The listing builds one solid part. Answer for the finished solid, in the listing's coordinates (mm). Face numbers are marked on the shaded views. A direction names the side the tool comes from. Coordinates: 2 decimals unless noted, no trailing zeros. Write each loop counter-clockwise with the first axis right and the second up, starting at its lowest first coordinate (ties: lowest second). Pieces come first, ordered by that corner, then holes.
(1) Which of the six approach directions +Z, -Z, +X, -X, +Y, -Y give full straight-line access (tool end or side, diameter ignored) to the marked faces 1, 2 and 3?
(2) Given P1, Ø5.5, axis at x = -24.892, y = 0, coming from the +Z side; P2, Ø9, axis at x = -25.4, y = 25.4, coming from the +Z side; P3, Ø4, axis at x = 36, z = 48.5, coming from the -Y side, each flat-ended and moving along its own axis, determine where each tip first touches the part or whether it passes through.
(3) The part is cut by section A-A on z = 8.5. Determine the outline of the cut face in (x, y).
(4) The part is cut by section C-C on z = 52.5. Determine the outline of the cut face in (x, y), plus the area to 3 significant figures.
(5) The part is cut by section B-B on x = 39.5. Determine the outline of the cut face in (y, z), plus the area to 3 significant figures.
(6) Straight lines are drawn through the part: line 1 (X direction, y = 25.4, z = 11.25); line 2 (Y direction, x = -25, z = 12); line 3 (Y direction, x = 28.5, z = 66). For each, find the intervals that lie inside material, in ascending order.
from build123d import *

# Parameters (mm, degrees)
F0_W     = 101.6
F0_H     = 76.2
F1_DEPTH = 25.4
F2_W     = 101.6
F2_H     = 33.5062108934
F3_DEPTH = 50.8
F4_R     = 1.0287
F5_DEPTH = 101.6
F6_R     = 3.0226
F6_R_2   = 1.0287
F7_DEPTH = 38.1


with BuildPart() as f1:
    # F0 (on Top) → F1 (new body)
    with BuildSketch(Plane.XY):
        Rectangle(F0_W, F0_H)
        with BuildLine():
            ThreePointArc((-25.4, 21.59), (-28.0940768363, 28.0940768363), (-21.59, 25.4))
            Line((-21.59, 25.4), (21.59, 25.4))
            ThreePointArc((21.59, 25.4), (25.4, 29.21), (29.21, 25.4))
            ThreePointArc((29.21, 25.4), (28.0940768363, 22.7059231637), (25.4, 21.59))
            Line((25.4, 21.59), (25.4, -21.59))
            ThreePointArc((25.4, -21.59), (28.0940768363, -22.7059231637), (29.21, -25.4))
            ThreePointArc((29.21, -25.4), (25.4, -29.21), (21.59, -25.4))
            Line((21.59, -25.4), (-21.59, -25.4))
            ThreePointArc((-21.59, -25.4), (-28.0940768363, -28.0940768363), (-25.4, -21.59))
            Line((-25.4, -21.59), (-25.4, 21.59))
        make_face(mode=Mode.SUBTRACT)
        with BuildLine():
            Line((21.59, 25.4), (-21.59, 25.4))
            ThreePointArc((-21.59, 25.4), (-22.7059231637, 22.7059231637), (-25.4, 21.59))
            Line((-25.4, 21.59), (-25.4, -21.59))
            ThreePointArc((-25.4, -21.59), (-22.7059231637, -22.7059231637), (-21.59, -25.4))
            Line((-21.59, -25.4), (21.59, -25.4))
            ThreePointArc((21.59, -25.4), (22.7059231637, -22.7059231637), (25.4, -21.59))
            Line((25.4, -21.59), (25.4, 21.59))
            ThreePointArc((25.4, 21.59), (22.7059231637, 22.7059231637), (21.59, 25.4))
        make_face()
    extrude(amount=F1_DEPTH)

    # F2 (on face) → F3 (join)
    with BuildSketch(Plane.XY.offset(25.4)):
        Rectangle(F2_W, F2_H)
    extrude(amount=F3_DEPTH)

    # F4 (on face) → F5 (cut)
    with BuildSketch(Plane.XY.offset(76.2)):
        with Locations((-24.892, 0)):
            Circle(F4_R)
    extrude(amount=-F5_DEPTH, mode=Mode.SUBTRACT)

    # F6 (on face) → F7 (cut)
    with BuildSketch(Plane.XY.offset(76.2)):
        with Locations((-24.892, 0)):
            Circle(F6_R)
        with Locations((-24.892, 0)):
            Circle(F6_R_2, mode=Mode.SUBTRACT)
    extrude(amount=-F7_DEPTH, mode=Mode.SUBTRACT)


solid = f1.part
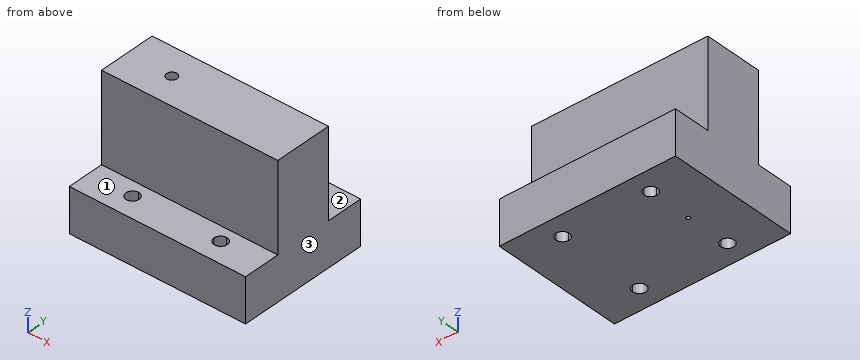
Model answer:
1. face 1: +Z, +X, -X, -Y
1. face 2: +Z, +X, -X, +Y
1. face 3: +Z, -Z, +X, +Y, -Y
2. P1: stops at z = 38.1
2. P2: stops at z = 25.4
2. P3: stops at y = -16.75
3. outline: (-50.8, -38.1) - (50.8, -38.1) - (50.8, 38.1) - (-50.8, 38.1) - close; hole circle Ø7.62 at (-25.4, -25.4); hole circle Ø7.62 at (-25.4, 25.4); hole circle Ø2.06 at (-24.89, 0); hole circle Ø7.62 at (25.4, -25.4); hole circle Ø7.62 at (25.4, 25.4)
4. outline: (-50.8, -16.75) - (50.8, -16.75) - (50.8, 16.75) - (-50.8, 16.75) - close; hole circle Ø6.05 at (-24.89, 0)
4. area: 3,380 mm2
5. outline: (-38.1, 0) - (38.1, 0) - (38.1, 25.4) - (16.75, 25.4) - (16.75, 76.2) - (-16.75, 76.2) - (-16.75, 25.4) - (-38.1, 25.4) - close
5. area: 3,640 mm2
6. line 1: x = -50.8 to -29.21, -21.59 to 21.59, 29.21 to 50.8
6. line 2: y = -38.1 to -29.19, -21.61 to -1.02, 1.02 to 21.61, 29.19 to 38.1
6. line 3: y = -16.75 to 16.75
